```python
from build123d import *

# Parameters (mm, degrees)
SKETCH1_W           = 63.5
SKETCH1_H           = 127
SKETCH1_R           = 12.7
SKETCH1_R_2         = 2.4892
BOSS_EXTRUDE1_DEPTH = 9.525
FILLET1_R           = 12.7


with BuildPart() as part:
    # Sketch1 → Boss-Extrude1 (new body)
    with BuildSketch(Plane(origin=(0, 0, 0), x_dir=(1, 0, 0), z_dir=(0, 1, 0))):
        with Locations((31.75, -63.5)):
            Rectangle(SKETCH1_W, SKETCH1_H)
        with Locations(Location((31.75, -25.4, 0), (0, 0, 90))):
            Circle(SKETCH1_R, mode=Mode.SUBTRACT)
        with Locations(Location((12.7, -114.3, 0), (0, 0, 90))):
            Circle(SKETCH1_R_2, mode=Mode.SUBTRACT)
        with Locations(Location((25.4, -114.3, 0), (0, 0, 90))):
            Circle(SKETCH1_R_2, mode=Mode.SUBTRACT)
        with Locations(Location((38.1, -114.3, 0), (0, 0, 90))):
            Circle(SKETCH1_R_2, mode=Mode.SUBTRACT)
        with Locations(Location((50.8, -114.3, 0), (0, 0, 90))):
            Circle(SKETCH1_R_2, mode=Mode.SUBTRACT)
    extrude(amount=BOSS_EXTRUDE1_DEPTH)

    # Fillet1
    fillet1_edges = [part.edges().sort_by_distance(p)[0] for p in [
        (0, 4.7625, 0),
        (63.5, 4.7625, 0),
        (63.5, 4.7625, 127),
        (0, 4.7625, 127),
    ]]
    fillet(fillet1_edges, radius=FILLET1_R)


solid = part.part
```
Can you work these out from the model? Positions are in its coordinate system, mm. Coordinates: 2 decimals unless noted, no trailing zeros. Loops run counter-clockwise (first coordinate to the right, second up) from the corner with the lowest first, then second, coordinate; pieces in that order, holes last. Notation, with made-up numbers: M -17,81 L 5,81 A10 cw 5,89 Z; hole C 38,46.5 d9. An arc over 180 degrees is marked long. Put each result on its own line as item: value. Start each with the question number.
(1) Imagine slicing it at B-B on y = 1.5. List the corners of the cut face in (x, z) for me.
(2) Imagine slicing it at A-A on x = 31.75. List the corners of the cut face in (y, z) for me (3 decimals).
(3) Imagine slicing it at D-D on x = 25.4. List the corners of the cut face in (y, z) for me (3 decimals).
(4) We'd pull the mould along X, two halves only. Please class faces 1 (the face through (53.23, 4.7, 114.84)), 2 (the face through (3.62, 4.83, 123.18)), 3 (the face through (31, 5, 127)): +X half, -X half, draft (parallel to the pull), parting line (faces both ways), or undercut.
(5) Imagine slicing it at C-C on z = 27.5. List the corners of the cut face in (x, y) for me (3 decimals), and give its area (3 significant figures).
(6) I need wall thicknesses on probe 1 along Z at (x, y) = (50.5, 6.75); probe 2 along X at (y, z) = (7.5, 25.4); probe 3 along Z at (x, y) = (25.4, 6). Which ranges of each line are inside material? Lowest first, please.
Worked answers:
1. outline: M 0,12.7 A12.7 ccw 12.7,0 L 50.8,0 A12.7 ccw 63.5,12.7 L 63.5,114.3 A12.7 ccw 50.8,127 L 12.7,127 A12.7 ccw 0,114.3 Z; hole C 12.7,114.3 d4.98; hole C 31.75,25.4 d25.4; hole C 25.4,114.3 d4.98; hole C 38.1,114.3 d4.98; hole C 50.8,114.3 d4.98
2. outline: M 0,0 L 9.525,0 L 9.525,12.7 L 0,12.7 Z; M 0,38.1 L 9.525,38.1 L 9.525,127 L 0,127 Z
3. outline: M 0,0 L 9.525,0 L 9.525,14.401 L 0,14.401 Z; M 0,36.399 L 9.525,36.399 L 9.525,111.811 L 0,111.811 Z; M 0,116.789 L 9.525,116.789 L 9.525,127 L 0,127 Z
4. face 1: undercut
4. face 2: -X half
4. face 3: draft
5. outline: M 0,0 L 19.225,0 L 19.225,9.525 L 0,9.525 Z; M 44.275,0 L 63.5,0 L 63.5,9.525 L 44.275,9.525 Z
5. area: 366 mm2
6. probe 1: z = 0 to 111.83, 116.77 to 127
6. probe 2: x = 0 to 19.05, 44.45 to 63.5
6. probe 3: z = 0 to 14.4, 36.4 to 111.81, 116.79 to 127
